```python
from build123d import *

# Parameters (mm, degrees)
CUT_EXTRUDE1_REACH = 14.9
SKETCH2_W          = 15
SKETCH2_H          = 1.85


with BuildPart() as part:
    # Sketch1 → Revolve1 (revolve)
    with BuildSketch(Plane(origin=(0, 0, 0), x_dir=(0, 0, -1), z_dir=(1, 0, 0))):
        Polygon((-7.5, 0), (-7.5, 1.85), (-5.85, 3.5), (-5.25, 3.5), (-10.9, 15.5), (-12.9, 15.5), (-12.9, 13.5), (-9.5, 6.278761062), (-9.5, 0), align=None)
    revolve(axis=Axis((0, 0, 0), (0, 1, 0)))

    # Sketch2 → Cut-Extrude1 (cut, up to next)
    with BuildSketch(Plane(origin=(0, 0, 0), x_dir=(0, 0, -1), z_dir=(1, 0, 0)), mode=Mode.PRIVATE) as cut_extrude1_sk1:
        with Locations((0, 0.925)):
            Rectangle(SKETCH2_W, SKETCH2_H)
    cut_extrude1_tool1 = extrude(cut_extrude1_sk1.sketch, amount=-CUT_EXTRUDE1_REACH, mode=Mode.PRIVATE) & part.part
    add(cut_extrude1_tool1.solids().sort_by_distance((0, 0.925, 0))[0], mode=Mode.SUBTRACT)


solid = part.part
```
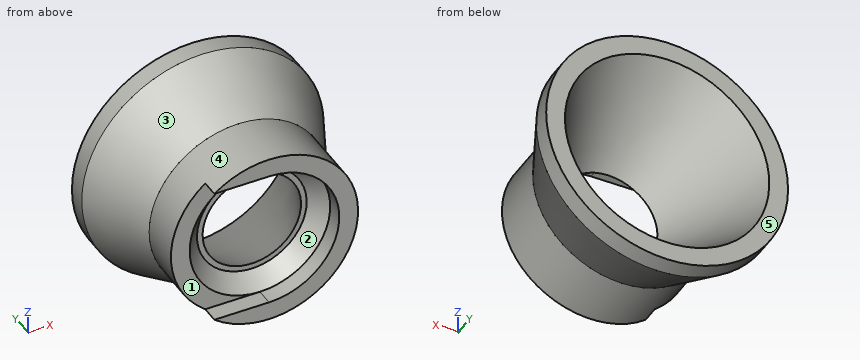
CAD build for the part. Positions are in the model's coordinates, mm. Face numbers are marked on the shaded views. A direction names the side the tool comes from. Give positions to 0.01 mm unless a question says otherwise; leave off trailing zeros. Loops run counter-clockwise (first coordinate to the right, second up) from the corner with the lowest first, then second, coordinate; pieces in that order, holes last. Notation, with made-up numbers: M 48,-2.75 L 99,-2.75 A14 cw 99,5.25 Z; hole C -13,-1.5 d11. An arc over 180 degrees is marked long. Use one line per item in the form item = value.
Item 1: Flat gauge pins, fed straight in: pin 1 (6 mm diameter, centred on x = 9.5, y = 10.5, fed in from +Z); pin 2 (0.6 mm diameter, centred on x = -3.5, y = 1, fed in from -Z); pin 3 (6 mm diameter, centred on x = 7, z = 3, fed in from -Y); pin 4 (6 mm diameter, centred on x = -9.5, z = -1.5, fed in from -Y). Where does each tip first touch, or does it go through?
Determined:
pin_1 = 10.09
pin_2 = -8.94
pin_3 = 0
pin_4 = 1.85
Item 2: Slice it at A-A (z = 0). List the corners of the cut face in (x, y).
Determined:
outline = M -12.9,13.5 L -9.5,6.28 L -9.5,1.85 L -7.5,1.85 L -5.85,3.5 L -5.25,3.5 L -10.9,15.5 L -12.9,15.5 Z; M 5.25,3.5 L 5.85,3.5 L 7.5,1.85 L 7.5,0 L 9.5,0 L 9.5,6.28 L 12.9,13.5 L 12.9,15.5 L 10.9,15.5 Z
Item 3: Two-plate mould, pull along X, no slides. Class the marked faces 1, 2 and 3: pulls with the +X half, pulls with the -X half, needs draft (parallel to the pull), parting line crosses it, or undercut.
Determined:
face_1 = needs draft
face_2 = undercut
face_3 = parting line crosses it
Item 4: Drill centre lines: probe 1 along X at (y, z) = (3.25, -4.75); probe 2 along Z at (x, y) = (-3.5, 13.5); probe 3 along X at (y, z) = (9, 3.5). Where is each one in solid material? Low to high. Write a range as from..to.
Determined:
probe_1 = -8.23..-3.83, 3.83..8.23
probe_2 = -12.42..-9.32, 9.32..12.42
probe_3 = -10.2..-7.01, 7.01..10.2
Item 5: Which spindle directions (+Z, -Z, +X, -X, +Y, -Y) get a long thin tool onto all of the face, cutting with end or side? Do the marked faces 4 and 5. Say none if no direction does.
Determined:
face_4 = -Y
face_5 = +Z, -Z, +X, -X, +Y
Item 6: Slice it at C-C (y = 7.25). List the corners of the cut face in (x, z), plus the area to 3 significant figures.
Determined:
outline = C 0,0 d19.91; hole C 0,0 d14.03
area = 157 mm2
Item 7: Slice it at B-B (y = 2.75). List the corners of the cut face in (x, z), plus the area to 3 significant figures.
Determined:
outline = C 0,0 d19; hole C 0,0 d13.2
area = 147 mm2
